The drawing under review shows one solid part. Ordinate dimensions are in mm from its lowest x, y, z. Coordinates: 2 decimals unless noted, no trailing zeros. Order: outer loops, then holes, each group sorted by start corner. A loop starts at its lowest first (then second) coordinate and runs counter-clockwise, first axis right, second up.
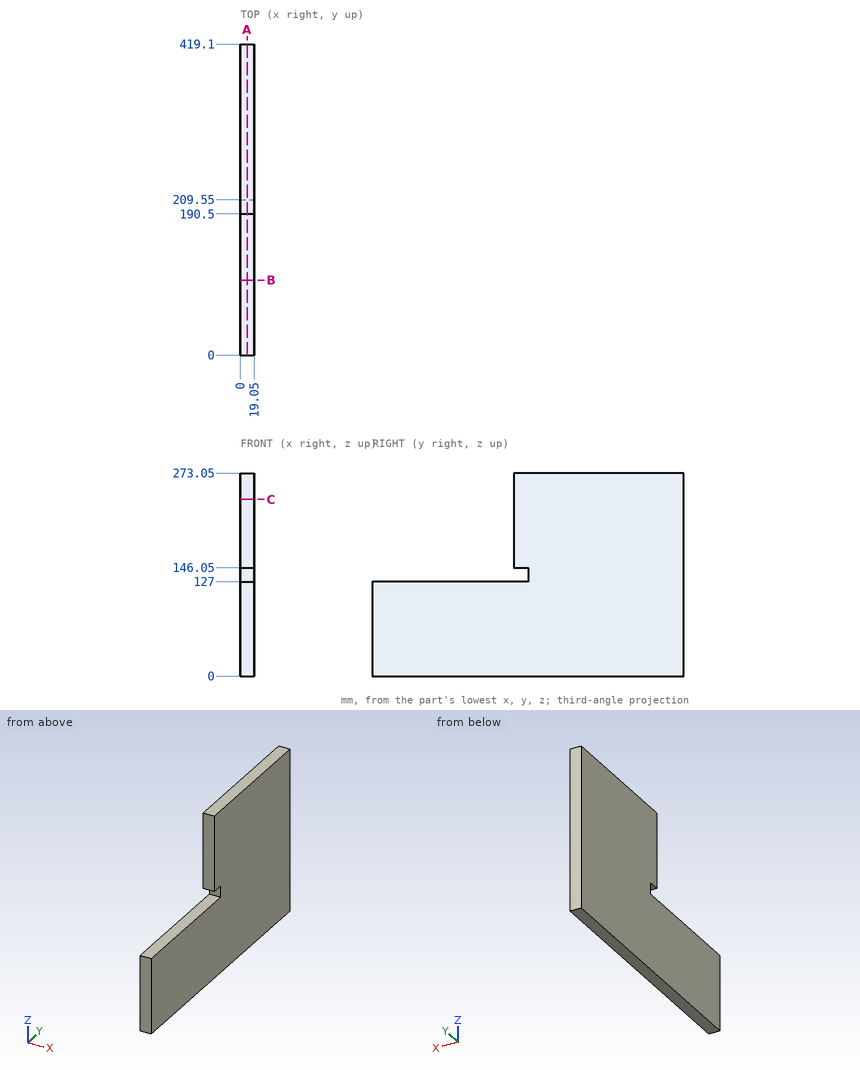
(1) Wall thickness on probe 1 along Y at (x, z) = (6.5, 192.5); probe 2 along Z at (x, y) = (1.5, 29.5): over which ranges is each line inside the solid? List them lowest first.
A:
probe 1: y = 190.5 to 419.1
probe 2: z = 0 to 127
(2) For pin 1 Ø8 at (x, z) = (7.5, 156) entering from -Y, flat-tipped, find the tip position at first contact; note if it passes through.
A:
pin 1: stops at y = 190.5
(3) We need section A-A, the plane x = 9.25. Write out the cut boundary in (y, z), and give its area (4 significant figures).
A:
outline: (0, 0) - (419.1, 0) - (419.1, 273.05) - (190.5, 273.05) - (190.5, 146.05) - (209.55, 146.05) - (209.55, 127) - (0, 127) - close
area: 86,250 mm2
(4) We need section C-C, the plane z = 238. Write out the cut boundary in (x, y).
A:
outline: (0, 190.5) - (19.05, 190.5) - (19.05, 419.1) - (0, 419.1) - close
(5) We need section B-B, the plane y = 101. Write out the cut boundary in (x, z).
A:
outline: (0, 0) - (19.05, 0) - (19.05, 127) - (0, 127) - close
